Design review of the part built by this model. Coordinates are the model's own, in mm. Face numbers are marked on the shaded views. Coordinates: 2 decimals unless noted, no trailing zeros. Loops run counter-clockwise (first coordinate to the right, second up) from the corner with the lowest first, then second, coordinate; pieces in that order, holes last. Notation, with made-up numbers: (-23, 24.25) -> (6, 24.25) arc R33 ccw to (6, 57.25) -> close; hole circle Ø9 at (8.25, -26.5). An arc over 180 degrees is marked (long way). Answer as a JSON object with one key per item and string values.
```python
from build123d import *

# Parameters (mm, degrees)
BOSS_EXTRUDE1_DEPTH = 80
SKETCH2_R           = 25
CUT_EXTRUDE1_DEPTH  = 50
SKETCH3_R           = 25
CUT_EXTRUDE2_DEPTH  = 80


with BuildPart() as part:
    # Sketch1 → Boss-Extrude1 (new body)
    with BuildSketch(Plane(origin=(0, 0, 0), x_dir=(1, 0, 0), z_dir=(0, 1, 0))):
        with BuildLine():
            Line((3.346152766, -99.944000629), (-296.48584912, -109.982458927))
            ThreePointArc((-296.48584912, -109.982458927), (-399.776002515, -13.384611064), (-303.178154652, 89.905542331))
            Line((-303.178154652, 89.905542331), (-3.346152766, 99.944000629))
            ThreePointArc((-3.346152766, 99.944000629), (99.944000629, 3.346152766), (3.346152766, -99.944000629))
        make_face()
    extrude(amount=BOSS_EXTRUDE1_DEPTH)

    # Sketch2 → Cut-Extrude1 (cut)
    with BuildSketch(Plane(origin=(0, 80, 0), x_dir=(1, 0, 0), z_dir=(0, 1, 0))):
        Circle(SKETCH2_R)
    extrude(amount=-CUT_EXTRUDE1_DEPTH, mode=Mode.SUBTRACT)

    # Sketch3 → Cut-Extrude2 (cut)
    with BuildSketch(Plane(origin=(0, 80, 0), x_dir=(1, 0, 0), z_dir=(0, 1, 0))):
        with Locations((-299.832001886, -10.038458298)):
            Circle(SKETCH3_R)
    extrude(amount=-CUT_EXTRUDE2_DEPTH, mode=Mode.SUBTRACT)


solid = part.part
```
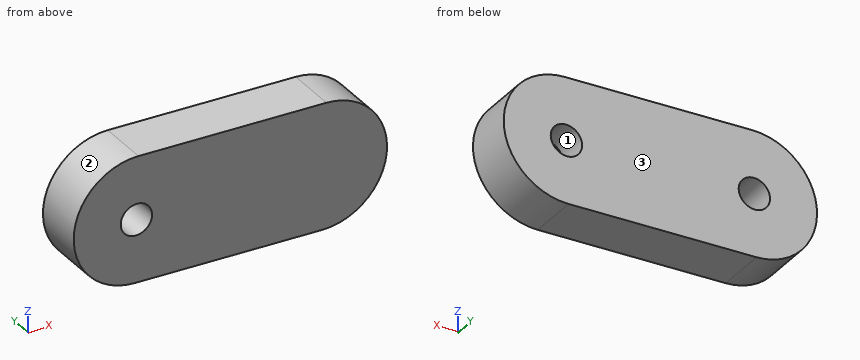
1) Clearance check with flat-ended pins moving along their axes: pin 1 Ø2 at (x, y) = (13.5, 20.5) entering from -Z; pin 2 Ø10 at (x, y) = (-190, 9) entering from -Z; pin 3 Ø12 at (x, z) = (-286.5, -44.5) entering from -Y; pin 4 Ø3 at (y, z) = (40.5, 46) entering from +X. State where each tip first meets the part, or that it passes through.
Completed:
{"pin 1": "z = -99.22", "pin 2": "z = -93.86", "pin 3": "y = 0", "pin 4": "x = 89.55"}
2) Add section A-A, the plane z = -8. Give the boundary of the cut face in (x, y), and give its area (3 significant figures).
Completed:
{"outline": "(-398.19, 0) -> (-317.14, 0) -> (-317.14, 80) -> (-398.19, 80) -> close; (-282.52, 0) -> (99.68, 0) -> (99.68, 80) -> (23.69, 80) -> (23.69, 30) -> (-23.69, 30) -> (-23.69, 80) -> (-282.52, 80) -> close", "area": "34,700 mm²"}
3) Add section C-C, the plane z = 29.5. Give the boundary of the cut face in (x, y), and give its area (3 significant figures).
Completed:
{"outline": "(-397.92, 0) -> (-315.52, 0) -> (-315.52, 80) -> (-397.92, 80) -> close; (-284.14, 0) -> (95.55, 0) -> (95.55, 80) -> (-284.14, 80) -> close", "area": "37,000 mm²"}
4) The part is to be moulded in two halves that separate along Z. For the marked faces 1, 2 and 3, say which applies: pulls with the +Z half, pulls with the -Z half, needs draft (parallel to the pull), parting line crosses it, or undercut.
Completed:
{"face 1": "undercut", "face 2": "parting line crosses it", "face 3": "needs draft"}
5) Add section D-D, the plane y = 10. Give the boundary of the cut face in (x, z), and give its area (3 significant figures).
Completed:
{"outline": "(-303.18, -89.91) -> (-3.35, -99.94) arc R100 ccw to (3.35, 99.94) -> (-296.49, 109.98) arc R100 ccw to start; hole circle Ø50 at (-299.83, 10.04)", "area": "89,500 mm²"}
6) Add section B-B, the plane y = 35. Give the boundary of the cut face in (x, z).
Completed:
{"outline": "(-303.18, -89.91) -> (-3.35, -99.94) arc R100 ccw to (3.35, 99.94) -> (-296.49, 109.98) arc R100 ccw to start; hole circle Ø50 at (-299.83, 10.04); hole circle Ø50 at (0, 0)"}
7) Wall thickness on probe 1 along X at (y, z) = (49, 0); probe 2 along X at (y, z) = (61.5, 12.5); probe 3 along Z at (x, y) = (3, 60): over which ranges is each line inside the solid? List them lowest first.
Completed:
{"probe 1": "-399.33 to -322.73, -276.94 to -25, 25 to 100", "probe 2": "-399.8 to -324.71, -274.95 to -21.65, 21.65 to 99.22", "probe 3": "-99.95 to -24.82, 24.82 to 99.96"}
